Build history of the part. All positions in model axes, mm. A direction names the side the tool comes from. Give positions to 0.01 mm unless a question says otherwise; leave off trailing zeros. Loops run counter-clockwise (first coordinate to the right, second up) from the corner with the lowest first, then second, coordinate; pieces in that order, holes last. Notation, with made-up numbers: M 3.25,10.5 L 59.25,10.5 A19 cw 59.25,27.5 Z; hole C 2,-35 d9. An arc over 180 degrees is marked long. Answer as a JSON object with one key per item and string values. Group by question number.
1. Slice it at A-A (z = -35.5). List the corners of the cut face in (x, y).
2. 3-axis set-ups, long thin cutter, end or side, ignore diameter. For faces 1 (the face through (7, 25, 1)), 2 (the face through (22, 12, -56)), 3 (the face through (12, -49, -4)), 4 (the face through (32.708, -1.352, -41.804)): which of +Z, -Z, +X, -X, +Y, -Y reach the whole face in a straight line?
3. Drill centre lines: line 1 along X through (y, z) = (20.5, 39.5); line 2 along X through (y, z) = (16.5, 39); line 3 along Y through (x, z) = (-37, -46). Where is each one in solid material? Low to high. Write a range as [from, to].
4. Mould opens along Y. For faces 5 (the face through (-7, 25, 1)), 6 (the face through (47.69, 15.02, 26.42)), 7 (the face through (22, 12, 56)), 8 (the face through (-0.96, -23.98, 0.78)) say: released by +Y, released by -Y, zero draft, split by the parting line, or undercut.
5. Drop flat-ended pins along their axis: pin 1 Ø4 at (y, z) = (26, -0.5) entering from -X; pin 2 Ø1 at (x, z) = (23.5, -13) entering from -Y; pin 3 Ø8 at (x, z) = (-40, 19) entering from -Y. Give the stop position or say it passes through.
from build123d import *

# Parameters (mm, degrees)
SKETCH1_R                  = 55
BOSS_EXTRUDE1_DEPTH        = 56
SKETCH2_R                  = 24
CUT_EXTRUDE1_DEPTH         = 112
SKETCH3_W                  = 14
SKETCH3_H                  = 7.6
CUT_EXTRUDE2_DEPTH         = 137.359818128
SKETCH4_OUTSIDE_W          = 150.338
SKETCH4_OUTSIDE_H          = 150.338
SKETCH4_OUTSIDE_R          = 50
CUT_EXTRUDE3_DEPTH         = 60
M10X1_0_TAPPED_HOLE1_D     = 9
M10X1_0_TAPPED_HOLE1_DEPTH = 28
M10X1_0_TAPPED_HOLE1_TIP   = 2.703872786


with BuildPart() as part:
    # Sketch1 → Boss-Extrude1 (new, symmetric)
    with BuildSketch(Plane.XY):
        Circle(SKETCH1_R)
    extrude(amount=BOSS_EXTRUDE1_DEPTH, both=True)

    # Sketch2 → Cut-Extrude1 (cut)
    with BuildSketch(Plane.XY.offset(56)):
        Circle(SKETCH2_R)
    extrude(amount=-CUT_EXTRUDE1_DEPTH, mode=Mode.SUBTRACT)

    # Sketch3 → Cut-Extrude2 (cut, through all)
    with BuildSketch(Plane.XY.offset(56)):
        with Locations((0, 24)):
            Rectangle(SKETCH3_W, SKETCH3_H)
    extrude(amount=-CUT_EXTRUDE2_DEPTH, mode=Mode.SUBTRACT)

    # Sketch4 outside → Cut-Extrude3 (cut)
    with BuildSketch(Plane.XY.offset(56)):
        Rectangle(SKETCH4_OUTSIDE_W, SKETCH4_OUTSIDE_H)
        Circle(SKETCH4_OUTSIDE_R, mode=Mode.SUBTRACT)
    extrude(amount=-CUT_EXTRUDE3_DEPTH, mode=Mode.SUBTRACT)

    # Sketch5 → Cut-Revolve1 (revolve, cut)
    with BuildSketch(Plane(origin=(0, 0, 0), x_dir=(1, 0, 0), z_dir=(0, 1, 0))):
        Polygon((50, 56), (55, 4), (55, 56), align=None)
    revolve(axis=Axis((0, 0, 0), (0, 0, -1)), mode=Mode.SUBTRACT)

    # M10x1.0 Tapped Hole1
    with Locations(Plane(origin=(-4.867734964, -29.256831772, -56), x_dir=(1, 0, 0), z_dir=(0, 0, -1))):
        with Locations((41.867734964, -29.256831772), (-32.132265036, -29.256831772)):
            Hole(M10X1_0_TAPPED_HOLE1_D / 2, depth=M10X1_0_TAPPED_HOLE1_DEPTH)
            with Locations((0, 0, -(M10X1_0_TAPPED_HOLE1_DEPTH + M10X1_0_TAPPED_HOLE1_TIP / 2))):  # 118° drill point
                Cone(0, M10X1_0_TAPPED_HOLE1_D / 2, M10X1_0_TAPPED_HOLE1_TIP, mode=Mode.SUBTRACT)


solid = part.part
Established:
{
 "1": {"outline": "C 0,0 d103.94; hole C -37,0 d9; hole M -7,22.96 A24 ccw long 7,22.96 L 7,27.8 L -7,27.8 Z; hole C 37,0 d9"},
 "2": {"face 1": "+Z, -Z", "face 2": "-Z, +X, -X, +Y, -Y", "face 3": "+Z", "face 4": "-Z"},
 "3": {"line 1": "x = [-45.6, -12.48], [12.48, 45.6]", "line 2": "x = [-47.2, -17.43], [17.43, 47.2]", "line 3": "y = [-35.04, -4.5], [4.5, 35.04]"},
 "4": {"face 5": "undercut", "face 6": "split by the parting line", "face 7": "zero draft", "face 8": "undercut"},
 "5": {"pin 1": "stops at x = -43.86", "pin 2": "stops at y = -49.01", "pin 3": "stops at y = -34.7"}
}
